Verification items for the finished model (mm, model axes). Coordinates: 2 decimals unless noted, no trailing zeros. Loops run counter-clockwise (first coordinate to the right, second up) from the corner with the lowest first, then second, coordinate; pieces in that order, holes last. Notation, with made-up numbers: (-37, 3.5) - (-22, 3.5) arc R29 ccw to (-22, 31.5) - close; hole circle Ø4 at (29.25, 53). An arc over 180 degrees is marked (long way). One line per item, written item: value. Start each with the question number.
(1) Section check B-B (x = -67). Record the boundary of the cut face in (y, z), plus the area to 3 significant figures.
(2) Section check A-A (z = 1.9). Record the boundary of the cut face in (x, y), plus the area to 3 significant figures.
(3) Thickness scan on probe 1 along Y at (x, z) = (70.5, 2.1); probe 2 along X at (y, z) = (-43.5, 1.4); probe 3 along Y at (x, z) = (-55, 2.5). Record the ranges inside material, lowest first. Write a range as [from, to].
(4) Section check C-C (y = 75). Record the boundary of the cut face in (x, z).
(5) Gauge pin test, flat end, axial feed: P1, Ø6, axis at x = -9.5, y = -23, coming from the -Z side. Record the tip position at first contact, or that the pin passes through.
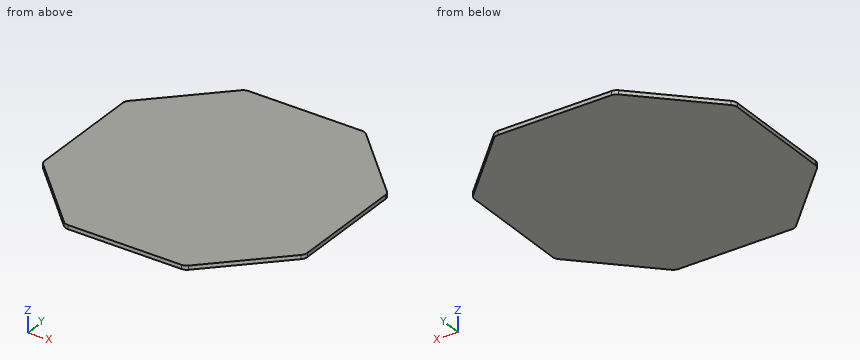
Autodesk Inventor part; units mm, degrees
ref_plane "YZ Plane" through (0, 0, 0) normal (1, 0, 0) x (0, 1, 0)
ref_plane "XZ Plane" through (0, 0, 0) normal (0, 1, 0) x (-1, 0, 0)
ref_plane "XY Plane" through (0, 0, 0) normal (0, 0, 1) x (1, 0, 0)
sketch "Sketch8" plane through (0, 0, 0) normal (0, 0, 1) x (1, 0, 0)
  line L0 (98.5, -98.5) -> (-98.5, -98.5)
  line L1 (-98.5, -98.5) -> (-98.5, 98.5)
  line L2 (-98.5, 98.5) -> (98.5, 98.5)
  line L3 (98.5, 98.5) -> (98.5, -98.5)
  line L4 (98.5, -98.5) -> (-98.5, 98.5) construction
  line L5 (-98.5, -98.5) -> (98.5, 98.5) construction
  line L6 (45, -98.5) -> (98.5, -45)
  line L7 (-45, -98.5) -> (-98.5, -45)
  line L8 (98.5, 45) -> (45, 98.5)
  line L9 (-45, 98.5) -> (-98.5, 45)
  line L10 (0, -98.5) -> (0, 98.5) construction
  point P0 (0, 0)
  dimension "d42" = 197
  dimension "d43" = 197
  dimension "d44" = 90
extrude "Plate3" add sketch "Sketch8" along normal blind 3 contours L0 L7 L1 L9 L2 L8 L3 L6
fillet "Corner Round1" radius 6 8 edges at (-45, -98.5, 1.5) (45, -98.5, 1.5) (98.5, -45, 1.5) (98.5, 45, 1.5) (45, 98.5, 1.5) (-45, 98.5, 1.5) (-98.5, 45, 1.5) (-98.5, -45, 1.5)
equation "\"d43\" = d42"
equation "\"d45\" = Thickness"
equation "\"BendReliefWidth\" = Thickness"
equation "\"BendReliefDepth\" = 0.5 * Thickness"
equation "\"CornerReliefSize\" = 4 * Thickness"
equation "\"MinimumRemnant\" = 2 * Thickness"
equation "\"TransitionRadius\" = BendRadius"
equation "\"JacobiRadiusSize\" = BendRadius"
equation "\"GapSize\" = Thickness"
properties part number "DSB 210 Axis cap" material "Stainless Steel"
Responses:
1. outline: (-76.5, 0) - (76.5, 0) - (76.5, 3) - (-76.5, 3) - close
1. area: 459 mm²
2. outline: (-98.5, -42.51) arc R6 ccw to (-96.74, -46.76) - (-46.76, -96.74) arc R6 ccw to (-42.51, -98.5) - (42.51, -98.5) arc R6 ccw to (46.76, -96.74) - (96.74, -46.76) arc R6 ccw to (98.5, -42.51) - (98.5, 42.51) arc R6 ccw to (96.74, 46.76) - (46.76, 96.74) arc R6 ccw to (42.51, 98.5) - (-42.51, 98.5) arc R6 ccw to (-46.76, 96.74) - (-96.74, 46.76) arc R6 ccw to (-98.5, 42.51) - close
2. area: 33,100 mm²
3. probe 1: y = [-73, 73]
3. probe 2: x = [-98.42, 98.42]
3. probe 3: y = [-88.5, 88.5]
4. outline: (-68.5, 0) - (68.5, 0) - (68.5, 3) - (-68.5, 3) - close
5. P1: stops at z = 0
